from build123d import *

# Parameters (mm, degrees)
SKETCH_1_W          = 76
SKETCH_1_H          = 50
EXTRUDE_1_DEPTH     = 12
SKETCH_2_R          = 3
CUT_EXTRUDE_1_DEPTH = 10
CUT_EXTRUDE_START   = -10
SKETCH_3_R          = 3
CUT_EXTRUDE_2_DEPTH = 10
SKETCH_4_R          = 3
CUT_EXTRUDE_3_DEPTH = 10
SKETCH_5_R          = 3
CUT_EXTRUDE_4_DEPTH = 12


with BuildPart() as part:
    # 草图1 → 凸台-拉伸1 (new body)
    with BuildSketch(Plane.XY):
        Rectangle(SKETCH_1_W, SKETCH_1_H)
    extrude(amount=EXTRUDE_1_DEPTH)

    # 草图2 → 切除-拉伸1 (cut)
    with BuildSketch(Plane.ZY.offset(38)):
        with Locations((6, -15)):
            Circle(SKETCH_2_R)
        with Locations((6, 0)):
            Circle(SKETCH_2_R)
        with Locations((6, 15)):
            Circle(SKETCH_2_R)
    extrude(amount=-CUT_EXTRUDE_1_DEPTH, mode=Mode.SUBTRACT)

    # 草图3 → 切除-拉伸2 (cut)
    with BuildSketch(Plane(origin=(38, 0, 0), x_dir=(0, 0, -1), z_dir=(1, 0, 0)).offset(CUT_EXTRUDE_START)):
        with Locations(Location((-6, -15, 0), (0, 0, 180))):
            Circle(SKETCH_3_R)
        with Locations(Location((-6, 0, 0), (0, 0, 180))):
            Circle(SKETCH_3_R)
        with Locations(Location((-6, 15, 0), (0, 0, 180))):
            Circle(SKETCH_3_R)
    extrude(amount=CUT_EXTRUDE_2_DEPTH, mode=Mode.SUBTRACT)

    # 草图4 → 切除-拉伸3 (cut)
    with BuildSketch(Plane.XZ.offset(25)):
        with Locations(Location((22.5, 6, 0), (0, 0, 270))):
            Circle(SKETCH_4_R)
        with Locations(Location((7.5, 6, 0), (0, 0, 270))):
            Circle(SKETCH_4_R)
        with Locations(Location((-7.5, 6, 0), (0, 0, 270))):
            Circle(SKETCH_4_R)
        with Locations(Location((-22.5, 6, 0), (0, 0, 270))):
            Circle(SKETCH_4_R)
    extrude(amount=-CUT_EXTRUDE_3_DEPTH, mode=Mode.SUBTRACT)

    # 草图5 → 切除-拉伸4 (cut)
    with BuildSketch(Plane(origin=(0, 0, 0), x_dir=(-1, 0, 0), z_dir=(0, 0, -1))):
        with Locations((0, -10)):
            Circle(SKETCH_5_R)
    extrude(amount=-CUT_EXTRUDE_4_DEPTH, mode=Mode.SUBTRACT)


solid = part.part
Input: part model. Units: mm. Frame: model coordinates. A direction names the side the tool comes from. Coordinates: 2 decimals unless noted, no trailing zeros. Loops run counter-clockwise (first coordinate to the right, second up) from the corner with the lowest first, then second, coordinate; pieces in that order, holes last.
(1) Section A-A on x = -33. Return the cut outline in (y, z).
(2) First-contact query: pin 1 Ø3.5 at (y, z) = (0, 6) entering from -X; pin 2 Ø3 at (x, z) = (-22.5, 5.5) entering from -Y; pin 3 Ø3.5 at (y, z) = (-15, 6) entering from +X. Flat tips, straight axial feed; report the tip coordinate or a pass-through.
(3) Pull-direction query (Y, two-part tool) for faces 1 (the face through (0, -7, 6)), 2 (the face through (28, 15, 6)), 3 (the face through (-38, 0, 2)), 4 (the face through (8, -15, 6)); classes: released by +Y, released by -Y, zero draft, split by the parting line, or undercut.
(4) Section B-B on y = 0. Return the cut outline in (x, z).
(5) Section C-C on x = -7.5. Return the cut outline in (y, z), then the cut area to 3 significant figures.
(6) Section D-D on y = 14. Return the cut outline in (x, z).
(7) Set-up query: faces 5 (the face through (38, 0, 2)), 6 (the face through (32.93, 17.93, 5.35)), 7 (the face through (-1, 25, 6)), 8 (the face through (-33.07, -1.15, 8.77)), 9 (the face through (-7, -15, 6)). Return all of +Z, -Z, +X, -X, +Y, -Y with unobstructed straight access to the full face (end or side cutting, diameter ignored); none if empty.
(8) Material intervals for probe 1 along X at (y, z) = (-21.25, 6); probe 2 along Y at (x, z) = (-31.5, 6); probe 3 along Y at (x, z) = (33, 4), sorted ascending.
Data:
1. outline: (-25, 0) - (25, 0) - (25, 12) - (-25, 12) - close; hole circle Ø6 at (-15, 6); hole circle Ø6 at (0, 6); hole circle Ø6 at (15, 6)
2. pin 1: stops at x = -28
2. pin 2: stops at y = -15
2. pin 3: stops at x = 28
3. face 1: undercut
3. face 2: undercut
3. face 3: zero draft
3. face 4: released by -Y
4. outline: (-38, 0) - (38, 0) - (38, 3) - (28, 3) - (28, 9) - (38, 9) - (38, 12) - (-38, 12) - (-38, 9) - (-28, 9) - (-28, 3) - (-38, 3) - close
5. outline: (-25, 0) - (25, 0) - (25, 12) - (-25, 12) - (-25, 9) - (-15, 9) - (-15, 3) - (-25, 3) - close
5. area: 540 mm2
6. outline: (-38, 0) - (38, 0) - (38, 3.17) - (28, 3.17) - (28, 8.83) - (38, 8.83) - (38, 12) - (-38, 12) - (-38, 8.83) - (-28, 8.83) - (-28, 3.17) - (-38, 3.17) - close
7. face 5: +Z, -Z, +X, +Y, -Y
7. face 6: +X
7. face 7: +Z, -Z, +X, -X, +Y
7. face 8: -X
7. face 9: -Y
8. probe 1: x = -38 to -25.5, -19.5 to -10.5, -4.5 to 4.5, 10.5 to 19.5, 25.5 to 38
8. probe 2: y = -25 to -18, -12 to -3, 3 to 12, 18 to 25
8. probe 3: y = -25 to -17.24, -12.76 to -2.24, 2.24 to 12.76, 17.24 to 25
